Part model, mm, in its own coordinate system. Face numbers are marked on the shaded views. A direction names the side the tool comes from. Coordinates: 2 decimals unless noted, no trailing zeros. Order: outer loops, then holes, each group sorted by start corner. A loop starts at its lowest first (then second) coordinate and runs counter-clockwise, first axis right, second up.
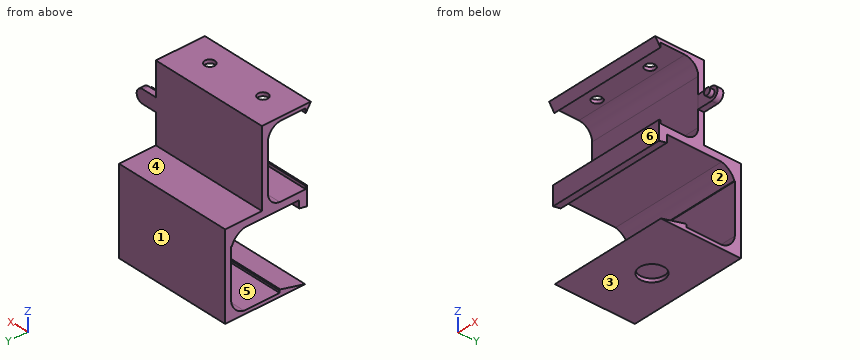
```python
from build123d import *

# Parameters (mm, degrees)
BOSS_EXTRUDE1_DEPTH      = 20
BOSS_EXTRUDE1_DEPTH_BACK = 20
BOSS_EXTRUDE2_DEPTH      = 2
SKETCH3_R                = 1.150002101
BOSS_EXTRUDE3_DEPTH      = 1.5
SKETCH4_R                = 4.175000755
CUT_EXTRUDE2_DEPTH       = 2
SKETCH5_R                = 1.705230735
SKETCH5_R_2              = 1.707530227
CUT_EXTRUDE4_DEPTH       = 2


with BuildPart() as part:
    # Sketch1 → Boss-Extrude1 (new, two sides: drawn at the far end of the back side and taken through both)
    with BuildSketch(Plane(origin=(0, 0, 0), x_dir=(0, 0, -1), z_dir=(1, 0, 0)).offset(-BOSS_EXTRUDE1_DEPTH_BACK)):
        with BuildLine():
            Line((-187.472492456, -316.815644503), (-187.472492456, -325.115650892))
            Line((-187.472492456, -325.115650892), (-185.972481966, -325.115650892))
            Line((-185.972481966, -325.115650892), (-188.672482967, -326.869040728))
            Line((-188.672482967, -326.869040728), (-188.672482967, -312.315642834))
            Line((-188.672482967, -312.315642834), (-188.672482967, -310.315638781))
            Line((-188.672482967, -310.315638781), (-162.915930152, -310.315638781))
            Line((-162.915930152, -310.315638781), (-162.915930152, -297.865658998))
            Line((-162.915930152, -297.865658998), (-134.240537882, -297.865658998))
            Line((-134.240537882, -297.865658998), (-134.240537882, -324.915647507))
            Line((-134.240537882, -324.915647507), (-136.367589235, -316.556811333))
            Line((-136.367589235, -316.556811333), (-136.14474237, -316.270142794))
            Line((-136.14474237, -316.270142794), (-135.440543294, -316.270142794))
            Line((-135.440543294, -316.270142794), (-135.440543294, -304.221749306))
            ThreePointArc((-135.440543294, -304.221749306), (-137.058677208, -301.304506823), (-140.081375837, -299.893140793))
            Line((-140.081375837, -299.893140793), (-156.763136387, -299.865663052))
            Line((-156.763136387, -299.865663052), (-156.763136387, -300.066769123))
            ThreePointArc((-156.763136387, -300.066769123), (-159.209325453, -301.733847579), (-160.555794835, -304.370135069))
            Line((-160.555794835, -304.370135069), (-160.555794835, -322.901427746))
            Line((-160.555794835, -322.901427746), (-158.084884286, -322.901427746))
            Line((-158.084884286, -322.901427746), (-157.503083348, -325.565636158))
            Line((-157.503083348, -325.565636158), (-162.915930152, -325.565636158))
            Line((-162.915930152, -325.565636158), (-163.915917277, -325.565636158))
            Line((-163.915917277, -325.565636158), (-163.915917277, -325.115650892))
            Line((-163.915917277, -325.115650892), (-162.915930152, -325.115650892))
            Line((-162.915930152, -325.115650892), (-162.940576673, -316.345274448))
            ThreePointArc((-162.940576673, -316.345274448), (-164.404833902, -313.471500259), (-167.41591692, -312.315642834))
            Line((-167.41591692, -312.315642834), (-182.972493545, -312.315642834))
            ThreePointArc((-182.972493545, -312.315642834), (-186.154473458, -313.633663782), (-187.472492456, -316.815644503))
        make_face()
    extrude(amount=BOSS_EXTRUDE1_DEPTH + BOSS_EXTRUDE1_DEPTH_BACK)

    # Sketch2 → Boss-Extrude2 (add)
    with BuildSketch(Plane(origin=(0, -310.315638781, 0), x_dir=(1, 0, 0), z_dir=(0, 1, 0))):
        with BuildLine():
            Line((19.999999553, -172.972485423), (25.000000373, -172.972485423))
            ThreePointArc((25.000000373, -172.972485423), (27.250001207, -175.222486258), (25.000000373, -177.472487092))
            Line((25.000000373, -177.472487092), (19.999999553, -177.472487092))
            Line((19.999999553, -177.472487092), (19.999999553, -172.972485423))
        make_face()
    extrude(amount=-BOSS_EXTRUDE2_DEPTH)


with BuildPart() as boss_extrude3_tool:
    # Sketch3 → Boss-Extrude3 (new body)
    with BuildSketch(Plane.XZ.offset(312.315642834)):
        with Locations(Location((25.000001633, 175.222481271, 0), (0, 0, 270))):
            Circle(SKETCH3_R)
    extrude(amount=BOSS_EXTRUDE3_DEPTH)


with BuildPart() as part_1:
    add(part.part)


with BuildPart() as part_2:
    # Boss-Extrude3: joined with boss_extrude3_tool
    add(part_1.part.fuse(boss_extrude3_tool.part, tol=0.00001))

    # Sketch4 → Cut-Extrude2 (cut)
    with BuildSketch(Plane(origin=(0, 0, 134.240537882), x_dir=(-1, 0, 0), z_dir=(0, 0, -1))):
        with Locations((-3.97e-07, -310.01564175)):
            Circle(SKETCH4_R)
    extrude(amount=-CUT_EXTRUDE2_DEPTH, mode=Mode.SUBTRACT)

    # Sketch5 → Cut-Extrude4 (cut)
    with BuildSketch(Plane.XY.offset(188.672482967)):
        with Locations((-10.003669951, -319.597688846)):
            Circle(SKETCH5_R)
        with Locations((9.993329109, -319.599979292)):
            Circle(SKETCH5_R_2)
    extrude(amount=-CUT_EXTRUDE4_DEPTH, mode=Mode.SUBTRACT)


solid = part_2.part
```
(1) Drop flat-ended pins along their axis: pin 1 (2.5 mm diameter, centred on x = 25, z = 175, fed in from -Y); pin 2 (1 mm diameter, centred on x = -0.5, z = 151, fed in from -Y); pin 3 (1.6 mm diameter, centred on x = 23, y = -311, fed in from -Z). Give the stop position or say it passes through.
(2) Tool access for the marked faces 4, 5 and 6: list every direction of +Z, -Z, +X, -X, +Y, -Y with a clear straight run to the whole face (end or side of a thin tool).
(3) Pull direction Y, two halves, no side cores. Call the marked faces 1, 2 and 3: +Y half, -Y half, draft (parallel to the pull), parting line (faces both ways), or undercut.
(4) Slice it at B-B, the plane x = -17. Give the cut face in (y, z), then the cut area to 3 significant figures.
(5) Probe line 1 (Z direction, x = 13.5, y = -304.75); line 2 (Z direction, x = 4.5, y = -313); line 3 (Z direction, x = 12, y = -321). List the from-to ranges inside material, lowest first.
Here are the results:
1. pin 1: stops at y = -313.82
1. pin 2: stops at y = -299.88
1. pin 3: stops at z = 172.97
2. face 4: +Z, +X, -X, +Y
2. face 5: +X, -X
2. face 6: -Z, +X, -X, -Y
3. face 1: +Y half
3. face 2: undercut
3. face 3: draft
4. outline: (-326.87, 188.67) - (-325.12, 185.97) - (-325.12, 187.47) - (-316.82, 187.47) arc R4.5 cw to (-312.32, 182.97) - (-312.32, 167.42) arc R4.5 cw to (-316.35, 162.94) - (-325.12, 162.92) - (-325.12, 163.92) - (-325.57, 163.92) - (-325.57, 157.5) - (-322.9, 158.08) - (-322.9, 160.56) - (-304.37, 160.56) arc R5.98 cw to (-300.07, 156.76) - (-299.87, 156.76) - (-299.89, 140.08) arc R5.4 cw to (-304.22, 135.44) - (-316.27, 135.44) - (-316.27, 136.14) - (-316.56, 136.37) - (-324.92, 134.24) - (-297.87, 134.24) - (-297.87, 162.92) - (-310.32, 162.92) - (-310.32, 188.67) - close
4. area: 245 mm2
5. line 1: z = 134.24 to 135.44, 160.56 to 162.92
5. line 2: z = 134.24 to 135.44, 160.56 to 165.03, 185.36 to 188.67
5. line 3: z = 134.24 to 135.24, 160.56 to 162.93, 187.47 to 188.67
